```python
from build123d import *

# Parameters (mm, degrees)
BOSS_EXTRUDE1_DEPTH  = 7
BOSS_EXTRUDE2_START  = 7
SKETCH1_3_W          = 3
SKETCH1_3_H          = 9
BOSS_EXTRUDE2_DEPTH  = 9
M3_CLEARANCE_HOLE1_D = 3.6
CHAMFER1_SIZE        = 2
CHAMFER1_SIZE2       = 2.856296013
FILLET1_R            = 10
FILLET2_R            = 2


with BuildPart() as part:
    # Sketch1 → Boss-Extrude1 (new body)
    with BuildSketch(Plane(origin=(0, 0, 0), x_dir=(1, 0, 0), z_dir=(0, 1, 0))):
        Polygon((-23.5, -9), (-23.5, 0), (23.5, 0), (23.5, -9), (26.5, -9), (26.5, 7), (15.5, 61), (15.5, 75), (12.5, 75), (12.5, 61), (11.415834914, 56), (21.397316395, 7), (21.397316395, 5), (-21.397316395, 5), (-21.397316395, 7), (-11.415834914, 56), (-12.5, 61), (-12.5, 75), (-15.5, 75), (-15.5, 61), (-26.5, 7), (-26.5, -9), align=None)
    extrude(amount=BOSS_EXTRUDE1_DEPTH)

    # Sketch1<3> → Boss-Extrude2 (add)
    with BuildSketch(Plane(origin=(0, 0, 0), x_dir=(1, 0, 0), z_dir=(0, 1, 0)).offset(BOSS_EXTRUDE2_START)):
        with Locations((-14, 70.5)):
            Rectangle(SKETCH1_3_W, SKETCH1_3_H)
        with Locations((14, 70.5)):
            Rectangle(SKETCH1_3_W, SKETCH1_3_H)
        with Locations((-25, -4.5)):
            Rectangle(SKETCH1_3_W, SKETCH1_3_H)
        with Locations((25, -4.5)):
            Rectangle(SKETCH1_3_W, SKETCH1_3_H)
    extrude(amount=BOSS_EXTRUDE2_DEPTH)

    # M3 Clearance Hole1 (through all)
    with Locations(Plane(origin=(26.5, 0, 0), x_dir=(0, 0, -1), z_dir=(1, 0, 0))):
        with Locations((-4.5, 11.5), (70.5, 11.5)):
            Hole(M3_CLEARANCE_HOLE1_D / 2)

    # Chamfer1
    chamfer1_edges = [part.edges().sort_by_distance(p)[0] for p in [
        (0, 7, 0),
    ]]
    chamfer1_side = [part.faces().sort_by_distance(p)[0] for p in [
        (0, 3.5, 0),
    ]]
    chamfer(chamfer1_edges, length=CHAMFER1_SIZE, length2=CHAMFER1_SIZE2, reference=chamfer1_side[0])

    # Fillet1
    # the kernel refuses this fillet: 10 mm, written as the material it adds along each edge
    with BuildSketch(Plane(origin=(-1.374685928, 7, 0), x_dir=(0, 0, -1), z_dir=(1, 0, 0))) as fillet1_piece_1_section:
        with BuildLine():
            CenterArc((9.949874371, 10), FILLET1_R, 185.739170477, 84.260829523)
            Line((0, 9), (0, 0))
            Line((0, 0), (9.949874371, 0))
        make_face()
    fillet1_piece_1 = extrude(amount=27.874685928, mode=Mode.PRIVATE)
    fillet1_piece_1 = split(fillet1_piece_1, bisect_by=Plane(origin=(10.011315234, 8.407248867, -4.866055679), z_dir=(0, -0.819152044288993, -0.5735764363510445)), keep=Keep.TOP, mode=Mode.PRIVATE)
    fillet1_piece_1 = split(fillet1_piece_1, bisect_by=Plane(origin=(10.011315234, 8.336481062, -5), z_dir=(0, 0, 1)), keep=Keep.TOP, mode=Mode.PRIVATE)
    add(fillet1_piece_1)
    with BuildSketch(Plane(origin=(-1.374685928, 7, 0), x_dir=(0, 0, -1), z_dir=(1, 0, 0))) as fillet1_piece_2_section:
        with BuildLine():
            CenterArc((9.949874371, 10), FILLET1_R, 185.739170477, 84.260829523)
            Line((0, 9), (0, 0))
            Line((0, 0), (9.949874371, 0))
        make_face()
    fillet1_piece_2 = extrude(amount=27.874685928, mode=Mode.PRIVATE)
    fillet1_piece_2 = split(fillet1_piece_2, bisect_by=Plane(origin=(26.506585427, 7.804991574, -6.967671542), z_dir=(-0.9798765487080173, 0, 0.19960448214422577)), keep=Keep.TOP, mode=Mode.PRIVATE)
    fillet1_piece_2 = split(fillet1_piece_2, bisect_by=Plane(origin=(21.601020113, 7.804991574, -5), z_dir=(0, 0, -1)), keep=Keep.TOP, mode=Mode.PRIVATE)
    fillet1_piece_2 = split(fillet1_piece_2, bisect_by=Plane(origin=(21.397316395, 7.804991574, -5.968389718), z_dir=(1, 0, 0)), keep=Keep.TOP, mode=Mode.PRIVATE)
    add(fillet1_piece_2)
    with BuildSketch(Plane(origin=(-1.374685928, 7, 0), x_dir=(0, 0, -1), z_dir=(1, 0, 0))) as fillet1_piece_3_section:
        with BuildLine():
            CenterArc((9.949874371, 10), FILLET1_R, 185.739170477, 84.260829523)
            Line((0, 9), (0, 0))
            Line((0, 0), (9.949874371, 0))
        make_face()
    fillet1_piece_3 = extrude(amount=52.749371855, mode=Mode.PRIVATE)
    fillet1_piece_3 = split(fillet1_piece_3, bisect_by=Plane(origin=(20.913958027, 7.01045348, -9.37285017), z_dir=(0.9798765487080173, 0, -0.1996044821442258)), keep=Keep.TOP, mode=Mode.PRIVATE)
    fillet1_piece_3 = split(fillet1_piece_3, bisect_by=Plane(origin=(21.397316395, 7.01045348, -9.450911129), z_dir=(-1, 0, 0)), keep=Keep.TOP, mode=Mode.PRIVATE)
    add(fillet1_piece_3)
    with BuildSketch(Plane(origin=(23.5, 7, 0), x_dir=(0, 0, -1), z_dir=(1, 0, 0))) as fillet1_piece_4_section:
        with BuildLine():
            CenterArc((9.949874371, 10), FILLET1_R, 185.739170477, 84.260829523)
            Line((0, 9), (0, 0))
            Line((0, 0), (9.949874371, 0))
        make_face()
    fillet1_piece_4 = extrude(amount=3, mode=Mode.PRIVATE)
    fillet1_piece_4 = split(fillet1_piece_4, bisect_by=Plane(origin=(25, 11.609815369, -5), z_dir=(0, 0, 1)), keep=Keep.TOP, mode=Mode.PRIVATE)
    add(fillet1_piece_4)
    with BuildSketch(Plane(origin=(-15.5, 7, -66), x_dir=(0, 0, 1), z_dir=(1, 0, 0))) as fillet1_piece_5_section:
        with BuildLine():
            CenterArc((9.949874371, -10), FILLET1_R, 90, 84.260829523)
            Line((0, -9), (0, 0))
            Line((0, 0), (9.949874371, 0))
        make_face()
    fillet1_piece_5 = extrude(amount=27.874685928, mode=Mode.PRIVATE)
    fillet1_piece_5 = split(fillet1_piece_5, bisect_by=Plane(origin=(-13.326382184, 11.537566275, -64.811145527), z_dir=(-0.9772894830316591, 0, 0.21190862737442448)), keep=Keep.TOP, mode=Mode.PRIVATE)
    add(fillet1_piece_5)
    with BuildSketch(Plane(origin=(-40.374685928, 7, -66), x_dir=(0, 0, 1), z_dir=(1, 0, 0))) as fillet1_piece_6_section:
        with BuildLine():
            CenterArc((9.949874371, -10), FILLET1_R, 90, 84.260829523)
            Line((0, -9), (0, 0))
            Line((0, 0), (9.949874371, 0))
        make_face()
    fillet1_piece_6 = extrude(amount=27.874685928, mode=Mode.PRIVATE)
    fillet1_piece_6 = split(fillet1_piece_6, bisect_by=Plane(origin=(-16.305903703, 7.017292707, -57.04374546), z_dir=(0.9798765487080173, 0, 0.19960448214422577)), keep=Keep.TOP, mode=Mode.PRIVATE)
    add(fillet1_piece_6)
    with BuildSketch(Plane(origin=(-40.374685928, 7, -66), x_dir=(0, 0, 1), z_dir=(1, 0, 0))) as fillet1_piece_7_section:
        with BuildLine():
            CenterArc((9.949874371, -10), FILLET1_R, 90, 84.260829523)
            Line((0, -9), (0, 0))
            Line((0, 0), (9.949874371, 0))
        make_face()
    fillet1_piece_7 = extrude(amount=52.749371855, mode=Mode.PRIVATE)
    fillet1_piece_7 = split(fillet1_piece_7, bisect_by=Plane(origin=(11.618519357, 7.008478839, -56.93474899), z_dir=(0.977289483031659, 0, 0.2119086273744248)), keep=Keep.TOP, mode=Mode.PRIVATE)
    add(fillet1_piece_7)
    with BuildSketch(Plane(origin=(-12.374685928, 7, -66), x_dir=(0, 0, 1), z_dir=(1, 0, 0))) as fillet1_piece_8_section:
        with BuildLine():
            CenterArc((9.949874371, -10), FILLET1_R, 90, 84.260829523)
            Line((0, -9), (0, 0))
            Line((0, 0), (9.949874371, 0))
        make_face()
    fillet1_piece_8 = extrude(amount=52.749371855, mode=Mode.PRIVATE)
    fillet1_piece_8 = split(fillet1_piece_8, bisect_by=Plane(origin=(-11.604329561, 7.008478839, -56.869307865), z_dir=(-0.9772894830316591, 0, 0.21190862737442448)), keep=Keep.TOP, mode=Mode.PRIVATE)
    add(fillet1_piece_8)
    with BuildSketch(Plane(origin=(12.5, 7, -66), x_dir=(0, 0, 1), z_dir=(1, 0, 0))) as fillet1_piece_9:
        with BuildLine():
            CenterArc((9.949874371, -10), FILLET1_R, 90, 84.260829523)
            Line((0, -9), (0, 0))
            Line((0, 0), (9.949874371, 0))
        make_face()
    extrude(amount=3)
    with BuildSketch(Plane(origin=(-12.374685928, 7, -66), x_dir=(0, 0, 1), z_dir=(1, 0, 0))) as fillet1_piece_10_section:
        with BuildLine():
            CenterArc((9.949874371, -10), FILLET1_R, 90, 84.260829523)
            Line((0, -9), (0, 0))
            Line((0, 0), (9.949874371, 0))
        make_face()
    fillet1_piece_10 = extrude(amount=52.749371855, mode=Mode.PRIVATE)
    fillet1_piece_10 = split(fillet1_piece_10, bisect_by=Plane(origin=(16.17255533, 7.017292707, -57.698364743), z_dir=(-0.9798765487080173, 0, 0.19960448214422577)), keep=Keep.TOP, mode=Mode.PRIVATE)
    fillet1_piece_10 = split(fillet1_piece_10, bisect_by=Plane(origin=(11.645733853, 7.017292707, -57.060257993), z_dir=(0.977289483031659, 0, 0.2119086273744248)), keep=Keep.TOP, mode=Mode.PRIVATE)
    add(fillet1_piece_10)
    with BuildSketch(Plane(origin=(1.374685928, 7, 0), x_dir=(0, 0, -1), z_dir=(-1, 0, 0))) as fillet1_piece_11_section:
        with BuildLine():
            CenterArc((9.949874371, -10), FILLET1_R, 90, 84.260829523)
            Line((0, -9), (0, 0))
            Line((0, 0), (9.949874371, 0))
        make_face()
    fillet1_piece_11 = extrude(amount=27.874685928, mode=Mode.PRIVATE)
    fillet1_piece_11 = split(fillet1_piece_11, bisect_by=Plane(origin=(-10.011315234, 8.407248867, -4.866055679), z_dir=(0, -0.819152044288993, -0.5735764363510445)), keep=Keep.TOP, mode=Mode.PRIVATE)
    fillet1_piece_11 = split(fillet1_piece_11, bisect_by=Plane(origin=(-10.011315234, 8.336481062, -5), z_dir=(0, 0, 1)), keep=Keep.TOP, mode=Mode.PRIVATE)
    add(fillet1_piece_11)
    with BuildSketch(Plane(origin=(1.374685928, 7, 0), x_dir=(0, 0, -1), z_dir=(-1, 0, 0))) as fillet1_piece_12_section:
        with BuildLine():
            CenterArc((9.949874371, -10), FILLET1_R, 90, 84.260829523)
            Line((0, -9), (0, 0))
            Line((0, 0), (9.949874371, 0))
        make_face()
    fillet1_piece_12 = extrude(amount=27.874685928, mode=Mode.PRIVATE)
    fillet1_piece_12 = split(fillet1_piece_12, bisect_by=Plane(origin=(-26.506585427, 7.804991574, -6.967671542), z_dir=(0.9798765487080173, 0, 0.19960448214422577)), keep=Keep.TOP, mode=Mode.PRIVATE)
    fillet1_piece_12 = split(fillet1_piece_12, bisect_by=Plane(origin=(-21.397316395, 7.804991574, -5.968389718), z_dir=(-1, 0, 0)), keep=Keep.TOP, mode=Mode.PRIVATE)
    fillet1_piece_12 = split(fillet1_piece_12, bisect_by=Plane(origin=(-21.601020113, 7.804991574, -5), z_dir=(0, 0, -1)), keep=Keep.TOP, mode=Mode.PRIVATE)
    add(fillet1_piece_12)
    with BuildSketch(Plane(origin=(1.374685928, 7, 0), x_dir=(0, 0, -1), z_dir=(-1, 0, 0))) as fillet1_piece_13_section:
        with BuildLine():
            CenterArc((9.949874371, -10), FILLET1_R, 90, 84.260829523)
            Line((0, -9), (0, 0))
            Line((0, 0), (9.949874371, 0))
        make_face()
    fillet1_piece_13 = extrude(amount=27.874685928, mode=Mode.PRIVATE)
    fillet1_piece_13 = split(fillet1_piece_13, bisect_by=Plane(origin=(-25.813340771, 7.01045348, -10.370872581), z_dir=(0.9798765487080173, 0, 0.19960448214422577)), keep=Keep.TOP, mode=Mode.PRIVATE)
    fillet1_piece_13 = split(fillet1_piece_13, bisect_by=Plane(origin=(-20.913958027, 7.01045348, -9.37285017), z_dir=(-0.9798765487080173, 0, -0.19960448214422577)), keep=Keep.TOP, mode=Mode.PRIVATE)
    fillet1_piece_13 = split(fillet1_piece_13, bisect_by=Plane(origin=(-21.297166367, 7.01045348, -5), z_dir=(0, 0, -1)), keep=Keep.TOP, mode=Mode.PRIVATE)
    add(fillet1_piece_13)
    with BuildSketch(Plane(origin=(-23.5, 7, 0), x_dir=(0, 0, -1), z_dir=(-1, 0, 0))) as fillet1_piece_14_section:
        with BuildLine():
            CenterArc((9.949874371, -10), FILLET1_R, 90, 84.260829523)
            Line((0, -9), (0, 0))
            Line((0, 0), (9.949874371, 0))
        make_face()
    fillet1_piece_14 = extrude(amount=3, mode=Mode.PRIVATE)
    fillet1_piece_14 = split(fillet1_piece_14, bisect_by=Plane(origin=(-25, 11.609815369, -5), z_dir=(0, 0, 1)), keep=Keep.TOP, mode=Mode.PRIVATE)
    add(fillet1_piece_14)

    # Fillet2
    fillet2_edges = [part.edges().sort_by_distance(p)[0] for p in [
        (25, 16, 9),
        (25, 16, 0),
        (-14, 16, -75),
        (-14, 16, -66),
        (14, 16, -75),
        (14, 16, -66),
        (-25, 16, 9),
        (-25, 16, 0),
    ]]
    fillet(fillet2_edges, radius=FILLET2_R)


solid = part.part
```
Work out the finished part from the listing and answer in its coordinate system (mm). A direction names the side the tool comes from. Round coordinates to 2 decimals unless told otherwise and drop trailing zeros. Loops run counter-clockwise (first coordinate to the right, second up) from the corner with the lowest first, then second, coordinate; pieces in that order, holes last. Notation, with made-up numbers: M 33,83.25 L 42,83.25 A25 cw 42,102.25 Z; hole C -8,54 d8. An arc over 180 degrees is marked long. One line per question, with ' | ' between items.
Q1. The mould has two halves that part along Z. Classify faces 1 (the flat face through (21, 3, -34)), 2 (the cylindrical face through (-14.02, 11.58, -72.3)), 3 (the cylindrical face through (24.979, 12.041, 6.217)), 4 (the flat face through (-25, 16, 4)): +Z half, -Z half, draft (parallel to the pull), parting line (faces both ways), or undercut.
Conclusion:
face 1: -Z half | face 2: undercut | face 3: undercut | face 4: draft
Q2. Each of these flat-tipped pins is pushed along its axis until it touches: pin 1 Ø2.5 at (x, y) = (3, 4.5) entering from -Z; pin 2 Ø4 at (x, y) = (-10.5, 2.5) entering from +Z; pin 3 Ø11.5 at (x, z) = (16.5, -26) entering from +Y; pin 4 Ø3 at (y, z) = (11.5, 4.5) entering from -X. Where does it stop, or does it pass through?
Conclusion:
pin 1: stops at z = -5 | pin 2: stops at z = 0 | pin 3: stops at y = 7 | pin 4: passes through
Q3. A tool of negligible diameter and unlimited length cuts with its end or side. For faces 5 (the flat face through (-19, 7, -33)), 6 (the flat face through (-21.397, 4, -6)), 7 (the flat face through (26.5, 6, 3)), from which of +Z, -Z, +X, -X, +Y, -Y can it reach the whole face along a straight path? Write none if from no direction.
Conclusion:
face 5: +X, -X, +Y | face 6: +Y, -Y | face 7: +Z, -Z, +X, +Y, -Y
Q4. Consider line 1 along Y through (x, z) = (14.5, -70.5); line 2 along X through (y, z) = (4.25, 4.5); line 3 along X through (y, z) = (7, -69). Determine where each line is inside the solid, lowest interval first. Write a range as from..to.
Conclusion:
line 1: y = 0..9.7, 13.3..16 | line 2: x = -26.5..-23.5, 23.5..26.5 | line 3: x = -15.5..-12.5, 12.5..15.5
Q5. Find section D-D, the plane y = 11.5. State how many separate pieces and enclosed holes the cut face has, then the cut area to 3 significant figures.
Conclusion:
separate pieces: 8 | enclosed holes: 0 | area: 84.0 mm2
Q6. Find section A-A, the plane z = 4.5. Give the vertices of the cut face in (x, y), then the cut area to 3 significant figures.
Conclusion:
outline: M -26.5,0 L -23.5,0 L -23.5,9.7 L -26.5,9.7 Z; M -26.5,13.3 L -23.5,13.3 L -23.5,16 L -26.5,16 Z; M 23.5,0 L 26.5,0 L 26.5,9.7 L 23.5,9.7 Z; M 23.5,13.3 L 26.5,13.3 L 26.5,16 L 23.5,16 Z | area: 74.4 mm2
Q7. Find section B-B, the plane x = -14. Give the vertices of the cut face in (y, z).
Conclusion:
outline: M 0,-75 L 14,-75 A2 ccw 16,-73 L 16,-67.67 A2 ccw 14.5,-65.73 A10 cw 7,-56.05 L 7,-43.31 L 0,-43.31 Z; M 0,-5 L 8.31,-5 A10 cw 8.4,-4.85 L 5,0 L 0,0 Z; hole C 11.5,-70.5 d3.6
Q8. Find section C-C, the plane z = -42. Give the vertices of the cut face in (x, y), then the cut area to 3 significant figures.
Conclusion:
outline: M -19.37,0 L -14.27,0 L -14.27,7 L -19.37,7 Z; M 14.27,0 L 19.37,0 L 19.37,7 L 14.27,7 Z | area: 71.4 mm2
